from build123d import *

# Parameters (mm, degrees)
F1_DEPTH       = 30
F3_DEPTH       = 27
F4_SIZE        = 2
F5_SIZE        = 2
F7_D           = 3.5
F7_CSINK_D     = 7
F7_CSINK_ANGLE = 90
F8_T1_DEPTH    = 108
F8_T6_DEPTH    = 25.6433659759
F8_T12_DEPTH   = 25.6433659759
F8_T17_DEPTH   = 25.6433659759
F8_T22_DEPTH   = 25.6433659759
F8_T26_ANGLE   = 90
F8_T28_ANGLE   = 90
F9_T1_DEPTH    = 100
F9_T6_DEPTH    = 40.0716830997
F9_T11_DEPTH   = 13.6286473502
F9_T17_DEPTH   = 13.6286473502
F9_T21_ANGLE   = 90
F9_T23_ANGLE   = 90
F9_T27_DEPTH   = 40.0716830997
F9_T33_DEPTH   = 13.6286473502
F9_T37_DEPTH   = 40.0716830997
F9_T44_DEPTH   = 40.0716830997
F9_T48_DEPTH   = 13.6286473502


# Not quite as in the source:
# - a fillet or chamfer that OpenCascade refuses, or shapes differently, is made with other operations: its cross-section is extruded or revolved along the edge and cut away or added


with BuildPart() as f1:
    # F0 (on Top) → F1 (new body)
    with BuildSketch(Plane.XY):
        with BuildLine():
            Line((-1.5, 0), (0, 0))
            Line((0, 0), (105, 0))
            Line((105, 0), (106.5, 0))
            ThreePointArc((106.5, 0), (112.1568542495, -2.3431457505), (114.5, -8))
            Line((114.5, -8), (114.5, -26.5))
            Line((114.5, -26.5), (94.5, -26.5))
            Line((94.5, -26.5), (94.5, -31.4999998882))
            Line((94.5, -31.4999998882), (115.4999998882, -31.4999998882))
            ThreePointArc((115.4999998882, -31.4999998882), (118.328427013, -30.328427013), (119.4999998882, -27.4999998882))
            Line((119.4999998882, -27.4999998882), (119.4999998882, 0.9999998882))
            ThreePointArc((119.4999998882, 0.9999998882), (118.328427013, 3.828427013), (115.4999998882, 4.9999998882))
            Line((115.4999998882, 4.9999998882), (109, 4.9999998882))
            Line((109, 4.9999998882), (105, 8.9999998882))
            Line((105, 8.9999998882), (105, 46.5))
            ThreePointArc((105, 46.5), (104.267766953, 48.267766953), (102.5, 49))
            Line((102.5, 49), (2.5, 49))
            ThreePointArc((2.5, 49), (0.732233047, 48.267766953), (0, 46.5))
            Line((0, 46.5), (0, 8.9999998882))
            Line((0, 8.9999998882), (-4, 4.9999998882))
            Line((-4, 4.9999998882), (-10.4999998882, 4.9999998882))
            ThreePointArc((-10.4999998882, 4.9999998882), (-13.328427013, 3.828427013), (-14.4999998882, 0.9999998882))
            Line((-14.4999998882, 0.9999998882), (-14.4999998882, -27.4999998882))
            ThreePointArc((-14.4999998882, -27.4999998882), (-13.328427013, -30.328427013), (-10.4999998882, -31.4999998882))
            Line((-10.4999998882, -31.4999998882), (10.5, -31.4999998882))
            Line((10.5, -31.4999998882), (10.5, -26.5))
            Line((10.5, -26.5), (-9.5, -26.5))
            Line((-9.5, -26.5), (-9.5, -8))
            ThreePointArc((-9.5, -8), (-7.1568542495, -2.3431457505), (-1.5, 0))
        make_face()
    extrude(amount=F1_DEPTH)

    # F2 (on face) → F3 (cut)
    with BuildSketch(Plane.XY.offset(30)):
        with BuildLine():
            Line((0, 0), (105, 0))
            Line((105, 0), (105, 4.9999998882))
            Line((105, 4.9999998882), (105, 8.9999998882))
            Line((105, 8.9999998882), (105, 46.5))
            ThreePointArc((105, 46.5), (104.267766953, 48.267766953), (102.5, 49))
            Line((102.5, 49), (2.5, 49))
            ThreePointArc((2.5, 49), (0.732233047, 48.267766953), (0, 46.5))
            Line((0, 46.5), (0, 8.9999998882))
            Line((0, 8.9999998882), (0, 4.9999998882))
            Line((0, 4.9999998882), (0, 0))
        make_face()
    extrude(amount=-F3_DEPTH, mode=Mode.SUBTRACT)

    # F4
    f4_edges = [f1.edges().sort_by_distance(p)[0] for p in [
        (94.5, -26.5, 15),
        (94.5, -31.5, 15),
        (10.5, -31.5, 15),
        (10.5, -26.5, 15),
    ]]
    chamfer(f4_edges, length=F4_SIZE)

    # F5
    f5_edges = [f1.edges().sort_by_distance(p)[0] for p in [
        (105.5, -26.5, 0),
        (-0.5, -26.5, 0),
        (-1, -31.5, 0),
        (106, -31.5, 0),
        (-7.25, 5, 30),
        (-9.5, -17.25, 30),
        (-0.5, -26.5, 30),
        (105.5, -26.5, 30),
        (106, -31.5, 30),
        (107, 7, 30),
        (-2, 7, 30),
    ]]
    chamfer(f5_edges, length=F5_SIZE)

    # F7 (through all)
    with Locations(Plane(origin=(0, 0, 0), x_dir=(1, 0, 0), z_dir=(0, 0, -1))):
        with Locations((6, -3.5), (6, -45.5), (99, -3.5), (99, -45.5)):
            CounterSinkHole(F7_D / 2, F7_CSINK_D / 2, counter_sink_angle=F7_CSINK_ANGLE)

    # F8: chamfer of 2 on 5 edges, made by hand

    # F8_s2 → F8_t1 (cut)
    with BuildSketch(Plane.YZ.offset(-1.5)):
        Polygon((2, 0), (0, 2), (0, 0), align=None)
    extrude(amount=F8_T1_DEPTH, mode=Mode.SUBTRACT)


with BuildPart() as f8_tool4:
    # F8_s5 → F8_t6 (new body)
    with BuildSketch(Plane.XZ.offset(33.6433659759)):
        Polygon((116.5, 0), (114.5, 2), (114.5, 0), align=None)
    extrude(amount=-F8_T6_DEPTH)

    split(bisect_by=Plane.XZ.offset(26.5), keep=Keep.TOP)

    split(bisect_by=Plane(origin=(0, -14.25, 14.25), x_dir=(1, 0, 0), z_dir=(0, 0.7071067812, -0.7071067812)), keep=Keep.TOP)


with BuildPart() as f1_1:
    add(f1.part)

    # F8_t3: cut F8_tool4
    add(f8_tool4.part, mode=Mode.SUBTRACT)


with BuildPart() as f8_tool10:
    # F8_s11 → F8_t12 (new body)
    with BuildSketch(Plane.XZ.offset(33.6433659759)):
        Polygon((116.5, 0), (114.5, 2), (114.5, 0), align=None)
    extrude(amount=-F8_T12_DEPTH)

    split(bisect_by=Plane.XZ.offset(26.5), keep=Keep.BOTTOM)


with BuildPart() as f1_2:
    add(f1_1.part)

    # F8_t9: cut F8_tool10
    add(f8_tool10.part, mode=Mode.SUBTRACT)


with BuildPart() as f8_tool15:
    # F8_s16 → F8_t17 (new body)
    with BuildSketch(Plane.XZ.offset(8)):
        Polygon((-11.5, 0), (-9.5, 2), (-9.5, 0), align=None)
    extrude(amount=F8_T17_DEPTH)

    split(bisect_by=Plane.XZ.offset(26.5), keep=Keep.BOTTOM)


with BuildPart() as f1_3:
    add(f1_2.part)

    # F8_t14: cut F8_tool15
    add(f8_tool15.part, mode=Mode.SUBTRACT)


with BuildPart() as f8_tool20:
    # F8_s21 → F8_t22 (new body)
    with BuildSketch(Plane.XZ.offset(8)):
        Polygon((-11.5, 0), (-9.5, 2), (-9.5, 0), align=None)
    extrude(amount=F8_T22_DEPTH)

    split(bisect_by=Plane.XZ.offset(26.5), keep=Keep.TOP)

    split(bisect_by=Plane(origin=(0, -14.25, 14.25), x_dir=(1, 0, 0), z_dir=(0, 0.7071067812, -0.7071067812)), keep=Keep.TOP)


with BuildPart() as f1_4:
    add(f1_3.part)

    # F8_t19: cut F8_tool20
    add(f8_tool20.part, mode=Mode.SUBTRACT)

    # F8_s25 → F8_t26 (revolve, cut)
    with BuildSketch(Plane.XZ.offset(8)):
        Polygon((-11.5, 0), (-9.5, 2), (-9.5, 0), align=None)
    revolve(axis=Axis((-1.5, -8, 0), (0, 0, -1)), revolution_arc=F8_T26_ANGLE, mode=Mode.SUBTRACT)

    # F8_s27 → F8_t28 (revolve, cut)
    with BuildSketch(Plane.YZ.offset(106.5)):
        Polygon((2, 0), (0, 2), (0, 0), align=None)
    revolve(axis=Axis((106.5, -8, 0), (0, 0, -1)), revolution_arc=F8_T28_ANGLE, mode=Mode.SUBTRACT)

    # F9: chamfer of 1 on 7 edges, made by hand

    # F9_s2 → F9_t1 (cut)
    with BuildSketch(Plane.YZ.offset(2.5)):
        Polygon((48, 0), (49, 1), (49, 0), align=None)
    extrude(amount=F9_T1_DEPTH, mode=Mode.SUBTRACT)


with BuildPart() as f9_tool4:
    # F9_s5 → F9_t6 (new body)
    with BuildSketch(Plane.XZ.offset(-46.5)):
        Polygon((1, 0), (0, 1), (0, 0), align=None)
    extrude(amount=F9_T6_DEPTH)

    split(bisect_by=Plane(origin=(-4.4999999441, 4.4999999441, 0), x_dir=(0, 0, 1), z_dir=(-0.7071067812, 0.7071067812, 0)), keep=Keep.TOP)


with BuildPart() as f1_5:
    add(f1_4.part)

    # F9_t3: cut F9_tool4
    add(f9_tool4.part, mode=Mode.SUBTRACT)


with BuildPart() as f9_tool9:
    # F9_s10 → F9_t11 (new body)
    with BuildSketch(Plane(origin=(-3.3184545357, -3.3184545357, 0), x_dir=(0, 0, 1), z_dir=(0.7071067812, 0.7071067812, 0))):
        Polygon((0, -5.3639609517), (1, -6.3639609517), (0, -6.3639609517), align=None)
    extrude(amount=F9_T11_DEPTH)

    split(bisect_by=Plane(origin=(0, 1.4999999441, -1.4999999441), x_dir=(1, 0, 0), z_dir=(0, 0.7071067812, -0.7071067812)), keep=Keep.TOP)

    split(bisect_by=Plane.YZ, keep=Keep.BOTTOM)


with BuildPart() as f1_6:
    add(f1_5.part)

    # F9_t8: cut F9_tool9
    add(f9_tool9.part, mode=Mode.SUBTRACT)


with BuildPart() as f9_tool15:
    # F9_s16 → F9_t17 (new body)
    with BuildSketch(Plane(origin=(46.181545576, -46.181545576, 0), x_dir=(0, 0, 1), z_dir=(0.7071067812, -0.7071067812, 0))):
        Polygon((0, -79.6101729762), (1, -80.6101729762), (0, -80.6101729762), align=None)
    extrude(amount=F9_T17_DEPTH)

    split(bisect_by=Plane.YZ.offset(105), keep=Keep.TOP)

    split(bisect_by=Plane(origin=(0, 1.4999999441, -1.4999999441), x_dir=(1, 0, 0), z_dir=(0, 0.7071067812, -0.7071067812)), keep=Keep.TOP)


with BuildPart() as f1_7:
    add(f1_6.part)

    # F9_t14: cut F9_tool15
    add(f9_tool15.part, mode=Mode.SUBTRACT)

    # F9_s20 → F9_t21 (revolve, cut)
    with BuildSketch(Plane.YZ.offset(2.5)):
        Polygon((48, 0), (49, 1), (49, 0), align=None)
    revolve(axis=Axis((2.5, 46.5, 0), (0, 0, 1)), revolution_arc=F9_T21_ANGLE, mode=Mode.SUBTRACT)

    # F9_s22 → F9_t23 (revolve, cut)
    with BuildSketch(Plane.XZ.offset(-46.5)):
        Polygon((104, 0), (105, 1), (105, 0), align=None)
    revolve(axis=Axis((102.5, 46.5, 0), (0, 0, 1)), revolution_arc=F9_T23_ANGLE, mode=Mode.SUBTRACT)


with BuildPart() as f9_tool25:
    # F9_s26 → F9_t27 (new body)
    with BuildSketch(Plane.XZ.offset(-6.4283169003)):
        Polygon((104, 0), (105, 1), (105, 0), align=None)
    extrude(amount=-F9_T27_DEPTH)

    split(bisect_by=Plane(origin=(56.9999999441, 56.9999999441, 0), x_dir=(0, 0, 1), z_dir=(0.7071067812, 0.7071067812, 0)), keep=Keep.TOP)


with BuildPart() as f1_8:
    add(f1_7.part)

    # F9_t24: cut F9_tool25
    add(f9_tool25.part, mode=Mode.SUBTRACT)


with BuildPart() as f9_tool31:
    # F9_s32 → F9_t33 (new body)
    with BuildSketch(Plane(origin=(-3.3184545357, -3.3184545357, 0), x_dir=(0, 0, 1), z_dir=(0.7071067812, 0.7071067812, 0))):
        Polygon((0, -5.3639609517), (1, -6.3639609517), (0, -6.3639609517), align=None)
    extrude(amount=F9_T33_DEPTH)

    split(bisect_by=Plane.YZ, keep=Keep.TOP)


with BuildPart() as f9_tool35:
    # F9_s36 → F9_t37 (new body)
    with BuildSketch(Plane.XZ.offset(-46.5)):
        Polygon((1, 0), (0, 1), (0, 0), align=None)
    extrude(amount=F9_T37_DEPTH)

    split(bisect_by=Plane(origin=(-4.4999999441, 4.4999999441, 0), x_dir=(0, 0, 1), z_dir=(0.7071067812, -0.7071067812, 0)), keep=Keep.TOP)


with BuildPart() as f9_tool31_1:
    add(f9_tool31.part)

    # F9_t39: intersect F9_tool35
    add(f9_tool35.part, mode=Mode.INTERSECT)


with BuildPart() as f1_9:
    add(f1_8.part)

    # F9_t29: cut F9_tool31
    add(f9_tool31_1.part, mode=Mode.SUBTRACT)


with BuildPart() as f9_tool42:
    # F9_s43 → F9_t44 (new body)
    with BuildSketch(Plane.XZ.offset(-6.4283169003)):
        Polygon((104, 0), (105, 1), (105, 0), align=None)
    extrude(amount=-F9_T44_DEPTH)

    split(bisect_by=Plane(origin=(56.9999999441, 56.9999999441, 0), x_dir=(0, 0, 1), z_dir=(-0.7071067812, -0.7071067812, 0)), keep=Keep.TOP)


with BuildPart() as f9_tool46:
    # F9_s47 → F9_t48 (new body)
    with BuildSketch(Plane(origin=(46.181545576, -46.181545576, 0), x_dir=(0, 0, 1), z_dir=(0.7071067812, -0.7071067812, 0))):
        Polygon((0, -79.6101729762), (1, -80.6101729762), (0, -80.6101729762), align=None)
    extrude(amount=F9_T48_DEPTH)

    split(bisect_by=Plane.YZ.offset(105), keep=Keep.BOTTOM)


with BuildPart() as f9_tool42_1:
    add(f9_tool42.part)

    # F9_t50: intersect F9_tool46
    add(f9_tool46.part, mode=Mode.INTERSECT)


with BuildPart() as f1_10:
    add(f1_9.part)

    # F9_t40: cut F9_tool42
    add(f9_tool42_1.part, mode=Mode.SUBTRACT)


solid = f1_10.part
Source: CAD feature listing. Evaluate the final solid. Frame: model axes, mm. A direction names the side the tool comes from. Coordinates: 2 decimals unless noted, no trailing zeros. Loops run counter-clockwise (first coordinate to the right, second up) from the corner with the lowest first, then second, coordinate; pieces in that order, holes last. Notation, with made-up numbers: M 60.5,72.5 L 98.5,72.5 A20 cw 98.5,99.5 Z; hole C 79.5,-40 d9. An arc over 180 degrees is marked long. Answer in a Markdown table with one row per item.
Q1. Draft query along Y for faces 3 (the flat face through (119.5, -13, 15)), 4 (the conical face through (112.47, -1.89, 1.46)), 5 (the cylindrical face through (-13.297, 3.859, 14.818)). Return one class per face: pulls with the +Y half, pulls with the -Y half, needs draft (parallel to the pull), parting line crosses it, or undercut.
Answers below:
| item | result |
|---|---|
| face 3 | needs draft |
| face 4 | undercut |
| face 5 | pulls with the +Y half |
Q2. First-contact query: pin 1 (0.8 mm diameter, centred on y = -29, z = 19, fed in from +X); pin 2 (2 mm diameter, centred on y = 30.5, z = 1.5, fed in from -X); pin 3 (5 mm diameter, centred on x = 32.5, y = 33, fed in from +Z). Flat tips, straight axial feed; report the tip coordinate or a pass-through.
Answers below:
| item | result |
|---|---|
| pin 1 | stops at x = 119.35 |
| pin 2 | stops at x = 0 |
| pin 3 | stops at z = 3 |
Q3. Section A-A on z = 24.5. Return the cut outline in (x, y), plus the area to 3 significant figures.
Answers below:
| item | result |
|---|---|
| outline | M -14.5,-27.5 A4 ccw -10.5,-31.5 L 8.5,-31.5 L 10.5,-29.5 L 10.5,-28.5 L 8.5,-26.5 L -9.5,-26.5 L -9.5,-8 A8 cw -1.5,0 L 0,0 L 0,9 L -4,5 L -10.5,5 A4 ccw -14.5,1 Z; M 94.5,-29.5 L 96.5,-31.5 L 115.5,-31.5 A4 ccw 119.5,-27.5 L 119.5,1 A4 ccw 115.5,5 L 109,5 L 105,9 L 105,0 L 106.5,0 A8 cw 114.5,-8 L 114.5,-26.5 L 96.5,-26.5 L 94.5,-28.5 Z |
| area | 682 mm^2 |
Q4. Ray query, probe 1 along X at (y, z) = (45.5, 2.7); probe 2 along Y at (x, z) = (99, 2.15); probe 3 along Y at (x, z) = (107, 4). Return the intervals inside material, ascending. Write a range as from..to.
Answers below:
| item | result |
|---|---|
| probe 1 | x = 0..4.25, 7.75..97.25, 100.75..105 |
| probe 2 | y = -31.5..-26.5, 0..1.75, 5.25..43.75, 47.25..49 |
| probe 3 | y = -31.5..-26.5, -0.02..7 |
Q5. Set-up query: faces 1 (the cylindrical face through (-7.219, -2.406, 14.818)), 2 (the flat face through (106, -31.5, 15)). Return all of +Z, -Z, +X, -X, +Y, -Y with unobstructed straight access to the full face (end or side cutting, diameter ignored); none if empty.
Answers below:
| item | result |
|---|---|
| face 1 | +Z, -Z |
| face 2 | +Z, -Z, +X, -X, -Y |
Q6. Section C-C on x = 99. Return the cut outline in (y, z), plus the area to 3 significant figures.
Answers below:
| item | result |
|---|---|
| outline | M -31.5,2 L -29.5,0 L -28.5,0 L -26.5,2 L -26.5,28 L -28.5,30 L -29.5,30 L -31.5,28 Z; M 0,2 L 1,1 L 1.75,1.75 L 1.75,3 L 0,3 Z; M 5.25,1.75 L 7,0 L 42,0 L 43.75,1.75 L 43.75,3 L 5.25,3 Z; M 47.25,1.75 L 48.5,0.5 L 49,1 L 49,3 L 47.25,3 Z |
| area | 261 mm^2 |
Q7. Section B-B on y = -17.5. Return the cut outline in (x, z), plus the area to 3 significant figures.
Answers below:
| item | result |
|---|---|
| outline | M -14.5,2 L -12.5,0 L -11.5,0 L -9.5,2 L -9.5,28 L -11.5,30 L -12.5,30 L -14.5,28 Z; M 114.5,2 L 116.5,0 L 117.5,0 L 119.5,2 L 119.5,28 L 117.5,30 L 114.5,30 Z |
| area | 286 mm^2 |
Q8. Section D-D on y = 33. Return the cut outline in (x, z).
Answers below:
| item | result |
|---|---|
| outline | M 0,1 L 1,0 L 104,0 L 105,1 L 105,3 L 0,3 Z |
